from build123d import *

# Parameters (mm, degrees)
SKETCH1_W           = 135
SKETCH1_H           = 122
BOSS_EXTRUDE1_DEPTH = 5.7
HOLE_W              = 50
HOLE_H              = 80
CUT_EXTRUDE2_DEPTH  = 70
SCREW_LOCATIONS_R   = 0.5
CUT_EXTRUDE3_DEPTH  = 52
CUT_EXTRUDE4_DEPTH  = 5.7


with BuildPart() as part:
    # Sketch1 → Boss-Extrude1 (new body)
    with BuildSketch(Plane(origin=(0, 0, 0), x_dir=(0, 0, -1), z_dir=(1, 0, 0))):
        with Locations((67.5, 61)):
            Rectangle(SKETCH1_W, SKETCH1_H)
    extrude(amount=BOSS_EXTRUDE1_DEPTH)

    # Hole → Cut-Extrude2 (cut)
    with BuildSketch(Plane(origin=(0, 0, 0), x_dir=(0, 0, -1), z_dir=(1, 0, 0))):
        with Locations((55, 60)):
            Rectangle(HOLE_W, HOLE_H)
    extrude(amount=CUT_EXTRUDE2_DEPTH, mode=Mode.SUBTRACT)

    # Screw Locations → Cut-Extrude3 (cut)
    with BuildSketch(Plane(origin=(0, 0, 0), x_dir=(0, 0, -1), z_dir=(1, 0, 0))):
        with Locations((25.23, 104.17)):
            Circle(SCREW_LOCATIONS_R)
        with Locations((84.77, 104.17)):
            Circle(SCREW_LOCATIONS_R)
        with Locations((25.23, 15.83)):
            Circle(SCREW_LOCATIONS_R)
        with Locations((84.77, 15.83)):
            Circle(SCREW_LOCATIONS_R)
    extrude(amount=CUT_EXTRUDE3_DEPTH, mode=Mode.SUBTRACT)

    # Sketch4 → Cut-Extrude4 (cut)
    with BuildSketch(Plane(origin=(0, 0, 0), x_dir=(0, 0, -1), z_dir=(1, 0, 0))):
        Polygon((0, 116), (26.9, 116), (26.9, 121.8), (54.1, 121.8), (54.1, 116), (80.9, 116), (80.9, 121.8), (108.1, 121.8), (108.1, 116), (135, 116), (135, 130), (0, 130), align=None)
        Polygon((0, -8), (0, 6), (26.9, 6), (26.9, 0.2), (54.1, 0.2), (54.1, 6), (80.9, 6), (80.9, 0.2), (108.1, 0.2), (108.1, 6), (135, 6), (135, -8), align=None)
    extrude(amount=CUT_EXTRUDE4_DEPTH, mode=Mode.SUBTRACT)


solid = part.part
Design review of the part built by this model. Coordinates are the model's own, in mm. A direction names the side the tool comes from. Give positions to 0.01 mm unless a question says otherwise; leave off trailing zeros. Loops run counter-clockwise (first coordinate to the right, second up) from the corner with the lowest first, then second, coordinate; pieces in that order, holes last. Notation, with made-up numbers: (28.25, 61.5) -> (83.25, 61.5) arc R34 cw to (83.25, 98.5) -> close; hole circle Ø5 at (48.25, 42.25). An arc over 180 degrees is marked (long way). One line per question, with ' | ' between items. Start each with the question number.
(1) Insertion check: P1, Ø3, axis at x = 4, y = 2, coming from the -Z side; P2, Ø3, axis at x = 3, z = -20, coming from the -Y side. Each pin has a flat end and moves straight along its axis. Give the tip position at first contact, or say it passes through.
(2) Draft analysis for pull direction Y (two halves, no side actions). For faces 1 (the face through (3, 3, -80.9)), 2 (the face through (3, 0.2, -94)), 3 (the face through (3, 20, -55)), 4 (the face through (3, 100, -55)), state which applies: +Y half, -Y half, draft (parallel to the pull), parting line (faces both ways), or undercut.
(3) For line 1 (Y direction, x = 1.3, z = -25.23); line 2 (Y direction, x = 2.3, z = -84.77); line 3 (Z direction, x = 4, y = 104.17), list the stretches that pass through material, from the lowest coordinate up.
(4) We need section B-B (x = 3.8). State the section outline as (y, z) points.
(5) We need section C-C (z = -38). State the section outline as (x, y) points.
(6) We need section A-A (y = 45). State the section outline as (x, z) points, and give its area (4 significant figures).
(7) For faces 5 (the face through (3, 6, -121)), 6 (the face through (3, 119, -108.1)), 7 (the face through (3, 59, -30)), list the 3-axis set-ups (+Z, -Z, +X, -X, +Y, -Y) from which the entire face can be reached by the end or side of a thin tool; tool diameter is ignored.
The answers:
1) P1: stops at z = -108.1 | P2: stops at y = 6
2) face 1: draft | face 2: -Y half | face 3: undercut | face 4: undercut
3) line 1: y = 6 to 15.33, 16.33 to 103.67, 104.67 to 116 | line 2: y = 0.2 to 15.33, 16.33 to 103.67, 104.67 to 121.8 | line 3: z = -135 to -85.27, -84.27 to -25.73, -24.73 to 0
4) outline: (0.2, -108.1) -> (6, -108.1) -> (6, -135) -> (116, -135) -> (116, -108.1) -> (121.8, -108.1) -> (121.8, -80.9) -> (116, -80.9) -> (116, -54.1) -> (121.8, -54.1) -> (121.8, -26.9) -> (116, -26.9) -> (116, 0) -> (6, 0) -> (6, -26.9) -> (0.2, -26.9) -> (0.2, -54.1) -> (6, -54.1) -> (6, -80.9) -> (0.2, -80.9) -> close; hole circle Ø1 at (15.83, -84.77); hole circle Ø1 at (15.83, -25.23); hole (20, -80) -> (100, -80) -> (100, -30) -> (20, -30) -> close; hole circle Ø1 at (104.17, -84.77); hole circle Ø1 at (104.17, -25.23)
5) outline: (0, 0.2) -> (5.7, 0.2) -> (5.7, 20) -> (0, 20) -> close; (0, 100) -> (5.7, 100) -> (5.7, 121.8) -> (0, 121.8) -> close
6) outline: (0, -135) -> (5.7, -135) -> (5.7, -80) -> (0, -80) -> close; (0, -30) -> (5.7, -30) -> (5.7, 0) -> (0, 0) -> close | area: 484.5 mm^2
7) face 5: -Z, +X, -X, -Y | face 6: -Z, +X, -X, +Y | face 7: +X, -X
